Build history of the part. All positions in model axes, mm. Face numbers are marked on the shaded views. A direction names the side the tool comes from. Coordinates: 2 decimals unless noted, no trailing zeros. Order: outer loops, then holes, each group sorted by start corner. A loop starts at its lowest first (then second) coordinate and runs counter-clockwise, first axis right, second up. Notation, with made-up numbers: (76.25, 85) - (122.25, 85) arc R11 ccw to (122.25, 99) - close; hole circle Ø7 at (59.25, 58.5). An arc over 180 degrees is marked (long way). Write each question's results on one line, items separated by ' | '.
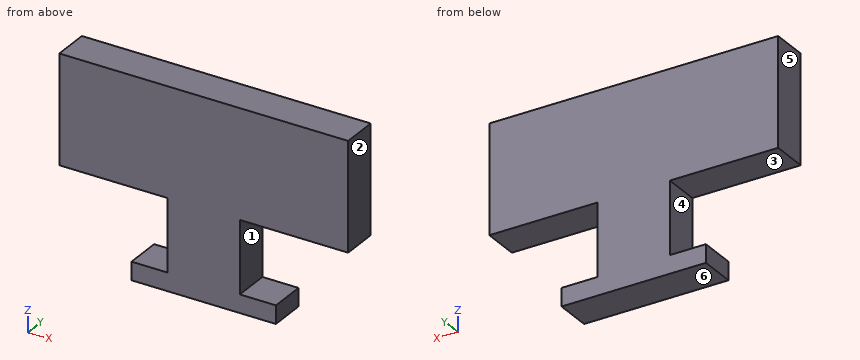
from build123d import *

# Parameters (mm, degrees)
F0_W     = 50.8
F0_H     = 50.8
F1_DEPTH = 25.4


with BuildPart() as f1:
    # F0 (on Front) → F1 (new body)
    with BuildSketch(Plane.XZ):
        Polygon((101.6, 38.1), (-101.6, 38.1), (-101.6, -38.1), (-25.4, -38.1), (25.4, -38.1), (101.6, -38.1), align=None)
        Polygon((25.4, -88.9), (-25.4, -88.9), (-50.8, -88.9), (-50.8, -101.6), (50.8, -101.6), (50.8, -88.9), align=None)
        with Locations((0, -63.5)):
            Rectangle(F0_W, F0_H)
    extrude(amount=F1_DEPTH)


solid = f1.part
1. Band-saw the part on B-B on z = -53. Give the cut face in (x, y), then the cut area to 3 significant figures.
Solved:
outline: (-25.4, -25.4) - (25.4, -25.4) - (25.4, 0) - (-25.4, 0) - close | area: 1,290 mm2
2. Tool access for the marked faces 1, 2 and 3: list every direction of +Z, -Z, +X, -X, +Y, -Y with a clear straight run to the whole face (end or side of a thin tool).
Solved:
face 1: +X, +Y, -Y | face 2: +Z, -Z, +X, +Y, -Y | face 3: -X, +Y, -Y
3. Band-saw the part on C-C on x = -61. Give the cut face in (y, z).
Solved:
outline: (-25.4, -38.1) - (0, -38.1) - (0, 38.1) - (-25.4, 38.1) - close
4. Probe line 1 (Z direction, x = 34, y = -5); line 2 (X direction, y = -8.5, z = -79); line 3 (X direction, y = -3.5, z = -95). List the from-to ranges inside material, lowest first.
Solved:
line 1: z = -101.6 to -88.9, -38.1 to 38.1 | line 2: x = -25.4 to 25.4 | line 3: x = -50.8 to 50.8
5. Band-saw the part on A-A on y = -16.25. Give the cut face in (x, z), then the cut area to 3 significant figures.
Solved:
outline: (-101.6, -38.1) - (-25.4, -38.1) - (-25.4, -88.9) - (-50.8, -88.9) - (-50.8, -101.6) - (50.8, -101.6) - (50.8, -88.9) - (25.4, -88.9) - (25.4, -38.1) - (101.6, -38.1) - (101.6, 38.1) - (-101.6, 38.1) - close | area: 19,400 mm2
6. Two-plate mould, pull along Z, no slides. Class the marked faces 4, 5 and 6: +Z half, -Z half, draft (parallel to the pull), parting line (faces both ways), or undercut.
Solved:
face 4: undercut | face 5: draft | face 6: -Z half
7. Drop flat-ended pins along their axis: pin 1 Ø10 at (y, z) = (-8.5, -93) entering from -X; pin 2 Ø10 at (y, z) = (-14, -95.5) entering from +X; pin 3 Ø12 at (y, z) = (-16.5, -72.5) entering from -X. Give the stop position or say it passes through.
Solved:
pin 1: stops at x = -50.8 | pin 2: stops at x = 50.8 | pin 3: stops at x = -25.4
